```python
from build123d import *

# Parameters (mm, degrees)
ESQUISSE2_R             = 50
BOSS_EXTRU_1_DEPTH      = 27
ESQUISSE3_R             = 32.2
ENL_V_MAT_EXTRU_1_DEPTH = 24
ESQUISSE4_R             = 32
BOSS_EXTRU_2_DEPTH      = 5
ESQUISSE5_R             = 29
ENL_V_MAT_EXTRU_2_DEPTH = 33
ESQUISSE6_R             = 4.25
ENL_V_MAT_EXTRU_3_DEPTH = 33
CHANFREIN1_SIZE         = 1


with BuildPart() as part:
    # Esquisse2 → Boss.-Extru.1 (new body)
    with BuildSketch(Plane.XY):
        Circle(ESQUISSE2_R)
    extrude(amount=BOSS_EXTRU_1_DEPTH)

    # Esquisse3 → Enlèv. mat.-Extru.1 (cut)
    with BuildSketch(Plane(origin=(0, 0, 0), x_dir=(-1, 0, 0), z_dir=(0, 0, -1))):
        Circle(ESQUISSE3_R)
    extrude(amount=-ENL_V_MAT_EXTRU_1_DEPTH, mode=Mode.SUBTRACT)

    # Esquisse4 → Boss.-Extru.2 (add)
    with BuildSketch(Plane.XY.offset(27)):
        Circle(ESQUISSE4_R)
    extrude(amount=BOSS_EXTRU_2_DEPTH)

    # Esquisse5 → Enlèv. mat.-Extru.2 (cut, through all)
    with BuildSketch(Plane.XY.offset(32)):
        Circle(ESQUISSE5_R)
    extrude(amount=-ENL_V_MAT_EXTRU_2_DEPTH, mode=Mode.SUBTRACT)

    # Esquisse6 → Enlèv. mat.-Extru.3 (cut, through all)
    with BuildSketch(Plane(origin=(0, 0, 0), x_dir=(-1, 0, 0), z_dir=(0, 0, -1))):
        with Locations((0, 40)):
            Circle(ESQUISSE6_R)
        with Locations((34.641016151, 20)):
            Circle(ESQUISSE6_R)
        with Locations((34.641016151, -20)):
            Circle(ESQUISSE6_R)
        with Locations((0, -40)):
            Circle(ESQUISSE6_R)
        with Locations((-34.641016151, -20)):
            Circle(ESQUISSE6_R)
        with Locations((-34.641016151, 20)):
            Circle(ESQUISSE6_R)
    extrude(amount=-ENL_V_MAT_EXTRU_3_DEPTH, mode=Mode.SUBTRACT)

    # Chanfrein1
    chanfrein1_edges = [part.edges().sort_by_distance(p)[0] for p in [
        (-32, 0, 32),
        (32.2, 0, 0),
    ]]
    chamfer(chanfrein1_edges, length=CHANFREIN1_SIZE)


solid = part.part
```
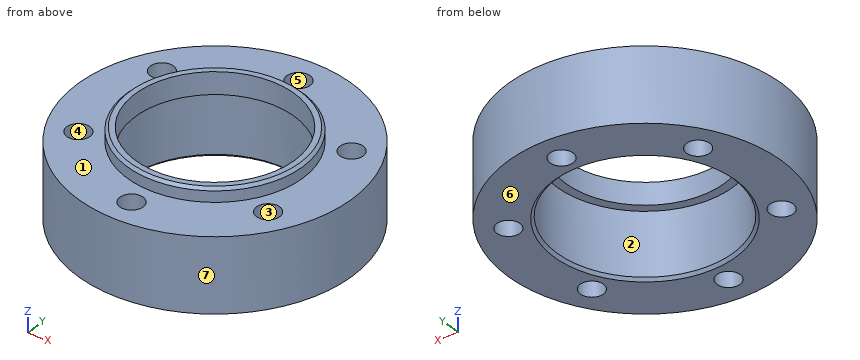
CAD build for the part. Positions are in the model's coordinates, mm. Face numbers are marked on the shaded views. A direction names the side the tool comes from. Round coordinates to 2 decimals unless told otherwise and drop trailing zeros. Order: outer loops, then holes, each group sorted by start corner. A loop starts at its lowest first (then second) coordinate and runs counter-clockwise, first axis right, second up.
Item 1: Probe line 1 along Y through (x, z) = (0, 19.75); line 2 along X through (y, z) = (-16.5, 17); line 3 along Y through (x, z) = (-35.5, 16). List the from-to ranges inside material, lowest first.
Item 2: Saw through at B-B on x = 0. Write the cut outline in (y, z), then the cut area to 3 significant figures.
Item 3: Mould opens along X. For the marked faces 4, 5, 6 and 7 say: pulls with the +X half, pulls with the -X half, needs draft (parallel to the pull), parting line crosses it, or undercut.
Item 4: Saw through at C-C on z = 5. Write the cut outline in (x, y), then the cut area to 3 significant figures.
Item 5: Saw through at D-D on y = 40. Write the cut outline in (x, z).
Item 6: Saw through at A-A on y = 0. Write the cut outline in (x, z).
Item 7: Pin check, flat tips, straight feed: pin 1 (12 mm diameter, centred on y = 29, z = 7.5, fed in from -X); pin 2 (6 mm diameter, centred on x = 39.5, y = -0.5, fed in from +Z); pin 3 (4 mm diameter, centred on x = -13, y = 30, fed in from -Z); pin 4 (1 mm diameter, centred on x = 32.5, y = 18, fed in from +Z). Stop position of each tip, or through.
Item 8: Tool access for the marked faces 1, 2 and 3: list every direction of +Z, -Z, +X, -X, +Y, -Y with a clear straight run to the whole face (end or side of a thin tool).
Reported:
1. line 1: y = -50 to -44.25, -35.75 to -32.2, 32.2 to 35.75, 44.25 to 50
1. line 2: x = -47.2 to -37.05, -32.23 to -27.65, 27.65 to 32.23, 37.05 to 47.2
1. line 3: y = -35.21 to -24.16, -15.84 to 15.84, 24.16 to 35.21
2. outline: (-50, 0) - (-44.25, 0) - (-44.25, 27) - (-50, 27) - close; (-35.75, 0) - (-33.2, 0) - (-32.2, 1) - (-32.2, 24) - (-29, 24) - (-29, 32) - (-31, 32) - (-32, 31) - (-32, 27) - (-35.75, 27) - close; (29, 24) - (32.2, 24) - (32.2, 1) - (33.2, 0) - (35.75, 0) - (35.75, 27) - (32, 27) - (32, 31) - (31, 32) - (29, 32) - close; (44.25, 0) - (50, 0) - (50, 27) - (44.25, 27) - close
2. area: 549 mm2
3. face 4: undercut
3. face 5: undercut
3. face 6: needs draft
3. face 7: parting line crosses it
4. outline: circle Ø100 at (0, 0); hole circle Ø8.5 at (-34.64, -20); hole circle Ø8.5 at (-34.64, 20); hole circle Ø64.4 at (0, 0); hole circle Ø8.5 at (0, -40); hole circle Ø8.5 at (0, 40); hole circle Ø8.5 at (34.64, -20); hole circle Ø8.5 at (34.64, 20)
4. area: 4,260 mm2
5. outline: (-30, 0) - (-4.25, 0) - (-4.25, 27) - (-30, 27) - close; (4.25, 0) - (30, 0) - (30, 27) - (4.25, 27) - close
6. outline: (-50, 0) - (-33.2, 0) - (-32.2, 1) - (-32.2, 24) - (-29, 24) - (-29, 32) - (-31, 32) - (-32, 31) - (-32, 27) - (-50, 27) - close; (29, 24) - (32.2, 24) - (32.2, 1) - (33.2, 0) - (50, 0) - (50, 27) - (32, 27) - (32, 31) - (31, 32) - (29, 32) - close
7. pin 1: stops at x = -44.4
7. pin 2: stops at z = 27
7. pin 3: stops at z = 0
7. pin 4: passes through
8. face 1: +Z
8. face 2: -Z
8. face 3: +Z, -Z
